Here's how the part is built. I have some questions about the finished solid (model axes, mm). Coordinates: 2 decimals unless noted, no trailing zeros. Loops run counter-clockwise (first coordinate to the right, second up) from the corner with the lowest first, then second, coordinate; pieces in that order, holes last. Notation, with made-up numbers: M 30,58 L 41,58 A19 cw 41,66 Z; hole C -35.75,36 d9. An arc over 180 degrees is marked long. Use CSV: the item, a comma, the result in double quotes. Start each with the question number.
Q1. If we section it at B-B (z = 2.9): Please give me the cut outline in (x, y).
Q2. If we section it at D-D (x = -179.5): Please give me the cut outline in (y, z).
Q3. Please list where these lines run through material, in increasing order: probe 1 along Y at (x, z) = (-10, 3.7); probe 2 along X at (y, z) = (7.5, 0.45); probe 3 along Y at (x, z) = (-85.5, 0.6). Write a range as [from, to].
Q4. If we section it at A-A (x = -210): Please give me the cut outline in (y, z), and give its area (3 significant figures).
Q5. If we section it at C-C (y = 7): Please give me the cut outline in (x, z).
Q6. For pin 1 Ø1.8 at (x, z) = (-108, 1.5) entering from -Y; pin 2 Ø1.8 at (y, z) = (-11, 2) entering from +X; pin 3 Ø1.4 at (y, z) = (-18, 4.5) entering from -X; pin 4 Ø10 at (x, y) = (-210, 10) entering from -Z, each with a flat end and sliding along its axis, tell me the tip position at first contact or that it passes through.
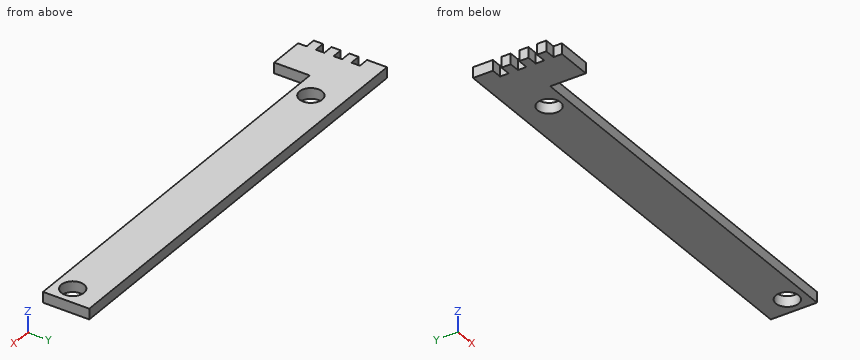
from build123d import *

# Parameters (mm, degrees)
ESQUISSE1_R        = 6.4
BOSS_EXTRU_1_DEPTH = 6


with BuildPart() as part:
    # Esquisse1 → Boss.-Extru.1 (new body)
    with BuildSketch(Plane.XY):
        Polygon((0, 0), (0, 26), (-250, 26), (-250, 20), (-250, 14.8), (-244, 14.8), (-244, 10), (-250, 10), (-250, 4.8), (-244, 4.8), (-244, 0), (-250, 0), (-250, -5.2), (-244, -5.2), (-244, -10), (-250, -10), (-250, -15.2), (-244, -15.2), (-244, -20), (-224, -20), (-224, 0), (-59.8, 0), align=None)
        with Locations((-210, 10)):
            Circle(ESQUISSE1_R, mode=Mode.SUBTRACT)
        with Locations((-10, 10)):
            Circle(ESQUISSE1_R, mode=Mode.SUBTRACT)
    extrude(amount=BOSS_EXTRU_1_DEPTH)


solid = part.part
Results below:
1,outline,"M -250,-15.2 L -244,-15.2 L -244,-20 L -224,-20 L -224,0 L 0,0 L 0,26 L -250,26 L -250,14.8 L -244,14.8 L -244,10 L -250,10 L -250,4.8 L -244,4.8 L -244,0 L -250,0 L -250,-5.2 L -244,-5.2 L -244,-10 L -250,-10 Z; hole C -210,10 d12.8; hole C -10,10 d12.8"
2,outline,"M 0,0 L 26,0 L 26,6 L 0,6 Z"
3,probe 1,"[0, 3.6], [16.4, 26]"
3,probe 2,"[-250, -215.89], [-204.11, -15.89], [-4.11, 0]"
3,probe 3,"[0, 26]"
4,outline,"M 0,0 L 3.6,0 L 3.6,6 L 0,6 Z; M 16.4,0 L 26,0 L 26,6 L 16.4,6 Z"
4,area,"79.2 mm^2"
5,outline,"M -250,0 L -215.65,0 L -215.65,6 L -250,6 Z; M -204.35,0 L -15.65,0 L -15.65,6 L -204.35,6 Z; M -4.35,0 L 0,0 L 0,6 L -4.35,6 Z"
6,pin 1,"y = 0"
6,pin 2,"x = -224"
6,pin 3,"x = -244"
6,pin 4,"through"
